For this review, take the finished solid that the model builds, in its own axes (mm). A direction names the side the tool comes from. Coordinates: 2 decimals unless noted, no trailing zeros. Write each loop counter-clockwise with the first axis right and the second up, starting at its lowest first coordinate (ties: lowest second). Pieces come first, ordered by that corner, then holes. Notation, with made-up numbers: M 75,51 L 121,51 A9 ccw 121,66 Z; hole C -4,-8.75 d4. An arc over 180 degrees is marked long. One line per question, with ' | ' between items.
from build123d import *

# Parameters (mm, degrees)
F1_W     = 254
F1_H     = 203.2
F2_DEPTH = 25.4
F3_DEPTH = 1019.048
F5_DEPTH = 103.124
F6_DEPTH = 72.898


with BuildPart() as f2:
    # F1 (on Top) → F2 (new body)
    with BuildSketch(Plane.XY):
        Rectangle(F1_W, F1_H)
    extrude(amount=-F2_DEPTH)

    # F0 (on Top) → F3 (join)
    with BuildSketch(Plane.XY):
        with BuildLine():
            ThreePointArc((57.15, 31.75), (55.2901280605, 36.2401280605), (50.8, 38.1))
            Line((50.8, 38.1), (-50.8, 38.1))
            ThreePointArc((-50.8, 38.1), (-55.2901280605, 36.2401280605), (-57.15, 31.75))
            ThreePointArc((-57.15, 31.75), (-55.2901280605, 27.2598719395), (-50.8, 25.4))
            Line((-50.8, 25.4), (-12.7, 25.4))
            ThreePointArc((-12.7, 25.4), (-8.2098719395, 23.5401280605), (-6.35, 19.05))
            Line((-6.35, 19.05), (-6.35, -19.05))
            ThreePointArc((-6.35, -19.05), (-8.2098719395, -23.5401280605), (-12.7, -25.4))
            Line((-12.7, -25.4), (-50.8, -25.4))
            ThreePointArc((-50.8, -25.4), (-55.2901280605, -27.2598719395), (-57.15, -31.75))
            ThreePointArc((-57.15, -31.75), (-55.2901280605, -36.2401280605), (-50.8, -38.1))
            Line((-50.8, -38.1), (50.8, -38.1))
            ThreePointArc((50.8, -38.1), (55.2901280605, -36.2401280605), (57.15, -31.75))
            ThreePointArc((57.15, -31.75), (55.2901280605, -27.2598719395), (50.8, -25.4))
            Line((50.8, -25.4), (12.7, -25.4))
            ThreePointArc((12.7, -25.4), (8.2098719395, -23.5401280605), (6.35, -19.05))
            Line((6.35, -19.05), (6.35, 19.05))
            ThreePointArc((6.35, 19.05), (8.2098719395, 23.5401280605), (12.7, 25.4))
            Line((12.7, 25.4), (50.8, 25.4))
            ThreePointArc((50.8, 25.4), (55.2901280605, 27.2598719395), (57.15, 31.75))
        make_face()
    extrude(amount=F3_DEPTH)

    # F4 (on Right) → F5 (cut, symmetric)
    with BuildSketch(Plane.YZ):
        with BuildLine():
            ThreePointArc((71.2698618146, 971.2817072868), (80.8566228106, 992.7335981743), (84.1375, 1016))
            ThreePointArc((84.1375, 1016), (-23.2664018257, 1096.8566228106), (-71.2698618146, 971.2817072868))
            ThreePointArc((-71.2698618146, 971.2817072868), (0, 931.8625), (71.2698618146, 971.2817072868))
        make_face()
    extrude(amount=F5_DEPTH, both=True, mode=Mode.SUBTRACT)

    # F4 (on Right) → F6 (join, symmetric)
    with BuildSketch(Plane.YZ):
        with BuildLine():
            ThreePointArc((71.2698618146, 971.2817072868), (0, 931.8625), (-71.2698618146, 971.2817072868))
            Line((-71.2698618146, 971.2817072868), (-89.4071367489, 971.2817072868))
            ThreePointArc((-89.4071367489, 971.2817072868), (0, 916.0331964859), (89.4071367489, 971.2817072868))
            Line((89.4071367489, 971.2817072868), (71.2698618146, 971.2817072868))
        make_face()
    extrude(amount=F6_DEPTH, both=True)


solid = f2.part
1. Take a section at A-A on y = -49. State the section outline as (x, z) points.
Computed values:
outline: M -127,-25.4 L 127,-25.4 L 127,0 L -127,0 Z; M -72.9,928.87 L 72.9,928.87 L 72.9,947.6 L -72.9,947.6 Z
2. Take a section at C-C on x = -103. State the section outline as (y, z) points, plus the area to 3 significant figures.
Computed values:
outline: M -101.6,-25.4 L 101.6,-25.4 L 101.6,0 L -101.6,0 Z | area: 5,160 mm2
3. Take a section at B-B on z = 781. State the section outline as (x, y) points, plus the area to 3 significant figures.
Computed values:
outline: M -50.8,-38.1 L 50.8,-38.1 A6.35 ccw 50.8,-25.4 L 12.7,-25.4 A6.35 cw 6.35,-19.05 L 6.35,19.05 A6.35 cw 12.7,25.4 L 50.8,25.4 A6.35 ccw 50.8,38.1 L -50.8,38.1 A6.35 ccw -50.8,25.4 L -12.7,25.4 A6.35 cw -6.35,19.05 L -6.35,-19.05 A6.35 cw -12.7,-25.4 L -50.8,-25.4 A6.35 ccw Z | area: 3,510 mm2
4. For line 1 along Y through (x, z) = (-18.5, 527.5); line 2 along Z through (x, y) = (44.5, 24); line 3 along Y through (x, z) = (-10.5, 18.5), list the stretches that pass through material, from the lowest coordinate up.
Computed values:
line 1: y = -38.1 to -25.4, 25.4 to 38.1 | line 2: z = -25.4 to 0, 918.96 to 935.36 | line 3: y = -38.1 to -25.01, 25.01 to 38.1
5. Take a section at D-D on y = -8.5. State the section outline as (x, z) points, plus the area to 3 significant figures.
Computed values:
outline: M -127,-25.4 L 127,-25.4 L 127,0 L 6.35,0 L 6.35,916.4 L 72.9,916.4 L 72.9,932.29 L -72.9,932.29 L -72.9,916.4 L -6.35,916.4 L -6.35,0 L -127,0 Z | area: 20,400 mm2
6. Clearance check with flat-ended pins moving along their axes: P1, Ø19, axis at x = 32, z = 539.5, coming from the -Y side; P2, Ø1.5, axis at x = 0.5, z = 438, coming from the +Y side; P3, Ø1.5, axis at y = -3.5, z = 227, coming from the +X side. State where each tip first meets the part, or that it passes through.
Computed values:
P1: stops at y = -38.1 | P2: stops at y = 38.1 | P3: stops at x = 6.35
7. Machinability: for faces 1 (the flat face through (6.35, 0, 453)), 2 (the flat face through (-31, -25.4, 453)), 3 (the flat face through (26, 1, 0)), which of the approach directions +Z, -Z, +X, -X, +Y, -Y give a long, thin tool a straight path to every point of the face, cutting with its end or side? Answer none if there is none.
Computed values:
face 1: +X | face 2: -X | face 3: none
8. Draft analysis for pull direction Y (two halves, no side actions). For faces 4 (the flat face through (-1, -38.1, 455)), 5 (the flat face through (127, -1, -13)), 6 (the flat face through (31, 25.4, 453)), 7 (the flat face through (1, 38.1, 455)), state which applies: pulls with the +Y half, pulls with the -Y half, needs draft (parallel to the pull), parting line crosses it, or undercut.
Computed values:
face 4: pulls with the -Y half | face 5: needs draft | face 6: undercut | face 7: pulls with the +Y half
